Read the model definition and answer for the solid it produces. Units are mm, in the model's axes. Give positions to 0.01 mm unless a question says otherwise; leave off trailing zeros. Loops run counter-clockwise (first coordinate to the right, second up) from the corner with the lowest first, then second, coordinate; pieces in that order, holes last. Notation, with made-up numbers: M -35.75,46 L 16.25,46 A12 ccw 16.25,51 Z; hole C 65.5,-6.5 d6. An arc over 180 degrees is marked long. Return JSON: item names as keys, results as strings. Group by question number.
```python
from build123d import *

# Parameters (mm, degrees)
F1_DEPTH = 25.4
F2_DEPTH = 25.4
F3_DEPTH = 25.4


with BuildPart() as f1:
    # F0 (on Right) → F1 (new body)
    with BuildSketch(Plane.YZ):
        Polygon((0, -12.8344558179), (61.9691237807, -12.8344558179), (81.6171616316, -12.8344558179), (132.2807371616, 47.9157753289), align=None)
    extrude(amount=F1_DEPTH)

    # F2 (add): a face of the model
    f2_faces = [f1.faces().sort_by_distance(p)[0] for p in [
        (25.4, 71.2992995977, 7.415621231),
    ]]
    extrude(f2_faces, amount=F2_DEPTH)

    # F3 (add): a face of the model
    f3_faces = [f1.faces().sort_by_distance(p)[0] for p in [
        (25.4, 66.1403685808, 17.5406597555),
    ]]
    extrude(f3_faces, amount=F3_DEPTH)


solid = f1.part
```
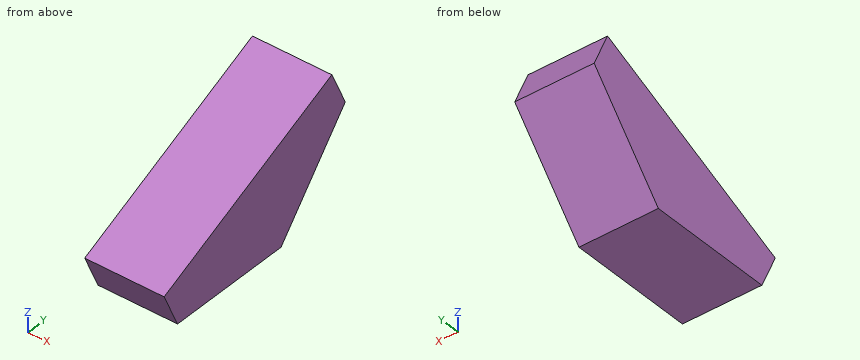
1. Straight lines are drawn through the part: line 1 along Z through (x, y) = (3, 10.5); line 2 along Z through (x, y) = (44, 5); line 3 along Y through (x, z) = (17.5, 19.5). For each, find the intervals that lie inside material, in ascending order.
2. Find section C-C (y = 69). Write down the section's boundary in (x, z).
3. Find section A-A (x = 12). Write down the section's boundary in (y, z).
4. Find section B-B (z = 4.5). Write down the section's boundary in (x, y), and give its area (3 significant figures).
5. Flat-ended cylindrical pins translate along their axes: P1, Ø12, axis at x = 39.5, z = 6.5, coming from the -Y side; P2, Ø4, axis at x = 18, z = 24.5, coming from the +Y side; P3, Ø1, axis at x = 34, z = 39.5, coming from the +Y side; P4, Ø1, axis at x = 44, y = 58.5, coming from the +Z side. Find the tip coordinate at first contact, or state that the pin passes through.
Result:
{
 "1": {"line 1": "z = -12.83 to 19.94", "line 2": "z = -12.83 to 17.41", "line 3": "y = 9.55 to 108.58"},
 "2": {"outline": "M 0,-12.83 L 50.8,-12.83 L 50.8,46.8 L 0,46.8 Z"},
 "3": {"outline": "M -10.6,10.25 L 0,-12.83 L 81.62,-12.83 L 132.28,47.92 L 121.68,71 Z"},
 "4": {"outline": "M 0,-7.96 L 50.8,-7.96 L 50.8,96.07 L 0,96.07 Z", "area": "5,280 mm2"},
 "5": {"P1": "stops at y = -10.6", "P2": "stops at y = 114.42", "P3": "stops at y = 125.68", "P4": "stops at z = 42.21"}
}
